The model under review builds one solid part; all positions refer to its coordinate system, in mm. A direction names the side the tool comes from. Coordinates: 2 decimals unless noted, no trailing zeros. Answer in a Markdown table with one row per item.
```python
from build123d import *

# Parameters (mm, degrees)
CUT_EXTRUDE1_DEPTH      = 19.7500001
CUT_EXTRUDE1_DEPTH_BACK = 19.7500001


with BuildPart() as part:
    # Sketch1 → Revolve1 (revolve)
    with BuildSketch(Plane(origin=(0, 0, 0), x_dir=(1, 0, 0), z_dir=(0, 1, 0))):
        with BuildLine():
            Line((18.75, -45.745065576), (18.75, -25.745065576))
            Line((18.75, -25.745065576), (4, -7))
            Line((4, -7), (4, -2))
            Line((4, -2), (0, -2))
            Line((0, -2), (0, -48.75))
            ThreePointArc((0, -48.75), (9.494631785, -47.99400364), (18.75, -45.745065576))
        make_face()
    revolve(axis=Axis((-21.521301372, 0, 0), (1, 0, 0)))

    # Mirror1: part across plane


with BuildPart() as part_1:
    add(part.part)
    add(part.part.mirror(Plane(origin=(0, 0, 2), x_dir=(0, 0, 1), z_dir=(-1, 0, 0))))

    # Sketch2 → Cut-Extrude1 (cut, two sides)
    with BuildSketch(Plane(origin=(0, 0, 0), x_dir=(0, 0, -1), z_dir=(1, 0, 0))) as cut_extrude1_sk:
        with BuildLine():
            ThreePointArc((-5.761847074, 3.975062049), (-4.114496766, 5.663118961), (-2, 6.708203932))
            Line((-2, 6.708203932), (-2, 21.652895347))
            ThreePointArc((-2, 21.652895347), (-12.781428856, 17.592127595), (-19.975093227, 8.593225672))
            Line((-19.975093227, 8.593225672), (-5.761847074, 3.975062049))
        make_face()
        with BuildLine():
            Line((2, 21.652895347), (2, 6.708203932))
            ThreePointArc((2, 6.708203932), (4.114496766, 5.663118961), (5.761847074, 3.975062049))
            Line((5.761847074, 3.975062049), (19.975093227, 8.593225672))
            ThreePointArc((19.975093227, 8.593225672), (12.781428856, 17.592127595), (2, 21.652895347))
        make_face()
        with BuildLine():
            Line((-14.345286543, -16.341989808), (-5.56101733, -4.251480479))
            ThreePointArc((-5.56101733, -4.251480479), (-6.657395614, -2.163118961), (-6.997915051, 0.170835984))
            Line((-6.997915051, 0.170835984), (-21.211161205, 4.788999607))
            ThreePointArc((-21.211161205, 4.788999607), (-20.680786313, -6.719594807), (-14.345286543, -16.341989808))
        make_face()
        with BuildLine():
            Line((21.211161205, 4.788999607), (6.997915051, 0.170835984))
            ThreePointArc((6.997915051, 0.170835984), (6.999478743, 0.085424353), (7, 0))
            ThreePointArc((7, 0), (6.630502293, -2.244201271), (5.56101733, -4.251480479))
            Line((5.56101733, -4.251480479), (14.345286543, -16.341989808))
            ThreePointArc((14.345286543, -16.341989808), (19.808925684, -8.969634338), (21.745065576, 0))
            ThreePointArc((21.745065576, 0), (21.611177296, 2.409334509), (21.211161205, 4.788999607))
        make_face()
        with BuildLine():
            Line((11.109218566, -18.693130818), (2.324949352, -6.602621488))
            ThreePointArc((2.324949352, -6.602621488), (0, -7), (-2.324949352, -6.602621488))
            Line((-2.324949352, -6.602621488), (-11.109218566, -18.693130818))
            ThreePointArc((-11.109218566, -18.693130818), (0, -21.745065576), (11.109218566, -18.693130818))
        make_face()
    extrude(amount=CUT_EXTRUDE1_DEPTH, mode=Mode.SUBTRACT)
    extrude(cut_extrude1_sk.sketch, amount=-CUT_EXTRUDE1_DEPTH_BACK, mode=Mode.SUBTRACT)


solid = part_1.part
```
Item 1: To check wall thickness, follow line 1 (Y direction, x = -1, z = 0); line 2 (Z direction, x = -6.5, y = 20); line 3 (Z direction, x = -2, y = -10.5). State the ranges of each line that lie inside material, in increasing order. Write a range as from..to.
Check values:
| item | result |
|---|---|
| line 1 | -48.74..-21.75, -7..-2, 2..48.74 |
| line 2 | -44.07..-8.54, -2..2, 8.54..44.07 |
| line 3 | -47.57..-19.04, -10.1..-5.16, 5.16..10.1, 19.04..47.57 |
Item 2: Clearance check with flat-ended pins moving along their axes: pin 1 Ø12 at (x, y) = (-9.5, 25) entering from +Z; pin 2 Ø7 at (y, z) = (-2.5, -2) entering from -X; pin 3 Ø4.5 at (x, y) = (2.5, 16) entering from -Z. State where each tip first meets the part, or that it passes through.
Check values:
| item | result |
|---|---|
| pin 1 | z = 44.24 |
| pin 2 | x = -4 |
| pin 3 | z = -46.72 |
Item 3: Mouldability with a two-part tool opening along Z and no side actions: class faces 4 (the face through (-18.75, 20, 20)), 5 (the face through (0.22, 6.83, 14.55)) as +Z half, -Z half, draft (parallel to the pull), parting line (faces both ways), or undercut.
Check values:
| item | result |
|---|---|
| face 4 | draft |
| face 5 | undercut |
Item 4: Tool access review of faces 1 (the face through (0.22, 2.96, 15.58)), 2 (the face through (-4, -2, 1)), 3 (the face through (4, -2, 1)): name each direction out of +Z, -Z, +X, -X, +Y, -Y from which nothing blocks a thin tool from reaching the whole face with its end or side.
Check values:
| item | result |
|---|---|
| face 1 | +X, -X |
| face 2 | -X |
| face 3 | +X |
Item 5: We need section A-A, the plane z = 0. State how many separate pieces and enclosed holes the cut face has, then the cut area to 3 significant figures.
Check values:
| item | result |
|---|---|
| separate pieces | 3 |
| enclosed holes | 0 |
| area | 2,290 mm^2 |
